Input: part model. Units: mm. Frame: model coordinates. A direction names the side the tool comes from. Coordinates: 2 decimals unless noted, no trailing zeros. Write each loop counter-clockwise with the first axis right and the second up, starting at its lowest first coordinate (ties: lowest second). Pieces come first, ordered by that corner, then holes. Notation, with made-up numbers: (10.5, -17.5) -> (52.5, -17.5) arc R7 cw to (52.5, -7.5) -> close; hole circle Ø9 at (36.5, 76.25). An arc over 180 degrees is marked (long way). Use one line per item in the form item = value. Start each with the question number.
(1) Cut plane D-D on y = 1.25. Return the cut outline in (x, z), plus the area to 3 significant figures.
(2) First-contact query: pin 1 (1 mm diameter, centred on y = -0.5, z = -0.5, fed in from -X); pin 2 (2 mm diameter, centred on y = -0.5, z = -1, fed in from +X). Flat tips, straight axial feed; report the tip coordinate or a pass-through.
(3) Pull-direction query (Y, two-part tool) for faces 1 (the face through (4, 0, -1.7)), 2 (the face through (1.5, -2.25, 0.5)), 3 (the face through (3, 1.75, 1)), 4 (the face through (2, 0, -2)); classes: released by +Y, released by -Y, zero draft, split by the parting line, or undercut.
(4) Cut plane C-C on x = 0.5. Return the cut outline in (y, z).
(5) Ray query, line 1 along Y through (x, z) = (2.05, 1.4); line 2 along Z through (x, y) = (2, 2); line 3 along Z through (x, y) = (3.15, -1.5). Return the intervals inside material, ascending.
(6) Cut plane B-B on x = 5.2. Return the cut outline in (y, z).
(7) Cut plane A-A on z = 0. State how many separate pieces and enclosed holes the cut face has, plus the area to 3 significant figures.
(8) Set-up query: faces 5 (the face through (1.2, 2, 0.6)), 6 (the face through (2, 0, 1.5)), 7 (the face through (1.5, -4.2, 0)). Return all of +Z, -Z, +X, -X, +Y, -Y with unobstructed straight access to the full face (end or side cutting, diameter ignored); none if empty.
```python
from build123d import *

# Parameters (mm, degrees)
SKETCH1_W               = 4
SKETCH1_H               = 4.5
SKETCH1_W_2             = 3
SKETCH1_H_2             = 3.5
BOSS_EXTRUDE1_DEPTH     = 4
SKETCH2_R               = 0.5
BOSS_EXTRUDE2_DEPTH     = 4.55
FILLET1_R               = 0.5
SKETCH3_R               = 1
CUT_EXTRUDE1_DEPTH      = 2.55
BOSS_EXTRUDE3_START     = -0.5
BOSS_EXTRUDE3_DEPTH     = 3
CUT_EXTRUDE2_DEPTH      = 1.5
SKETCH7_W               = 0.349986897
SKETCH7_H               = 2
CUT_EXTRUDE3_DEPTH      = 4.5
CUT_EXTRUDE3_DEPTH_BACK = 7.5


with BuildPart() as part:
    # Sketch1 → Boss-Extrude1 (new body)
    with BuildSketch(Plane(origin=(0, 0, 0), x_dir=(0, 0, -1), z_dir=(1, 0, 0))):
        Rectangle(SKETCH1_W, SKETCH1_H)
        Rectangle(SKETCH1_W_2, SKETCH1_H_2, mode=Mode.SUBTRACT)
    extrude(amount=BOSS_EXTRUDE1_DEPTH)

    # Sketch2 → Boss-Extrude2 (add)
    with BuildSketch(Plane.XZ.offset(2.25)):
        with Locations((2, 0)):
            Circle(SKETCH2_R)
    extrude(amount=BOSS_EXTRUDE2_DEPTH)

    # Fillet1
    fillet1_edges = [part.edges().sort_by_distance(p)[0] for p in [
        (1.5, -6.8, 0),
    ]]
    fillet(fillet1_edges, radius=FILLET1_R)

    # Sketch3 → Cut-Extrude1 (cut)
    with BuildSketch(Plane(origin=(0, 2.25, 0), x_dir=(1, 0, 0), z_dir=(0, 1, 0))):
        with Locations((2, 0)):
            Circle(SKETCH3_R)
    extrude(amount=-CUT_EXTRUDE1_DEPTH, mode=Mode.SUBTRACT)

    # Sketch5 → Boss-Extrude3 (add)
    with BuildSketch(Plane.XY.offset(2).offset(BOSS_EXTRUDE3_START)):
        with BuildLine():
            Line((4, 2.25), (4.403883865, 2.25))
            ThreePointArc((4.403883865, 2.25), (4.586458051, 2.215474668), (4.743818499, 2.116666667))
            Line((4.743818499, 2.116666667), (5.813186883, 1.125261165))
            ThreePointArc((5.813186883, 1.125261165), (5.973243782, 0.755684806), (5.808896382, 0.387996313))
            Line((5.808896382, 0.387996313), (4.596439486, -0.710104164))
            ThreePointArc((4.596439486, -0.710104164), (4.344752484, -0.832406779), (4.066768671, -0.800324431))
            Line((4.066768671, -0.800324431), (1.595431684, 0.240227029))
            Line((1.595431684, 0.240227029), (1.595431684, 0.359579889))
            Line((1.595431684, 0.359579889), (4.04486832, -0.671750473))
            ThreePointArc((4.04486832, -0.671750473), (4.322852132, -0.703832821), (4.574539135, -0.581530206))
            Line((4.574539135, -0.581530206), (5.646078544, 0.388943829))
            ThreePointArc((5.646078544, 0.388943829), (5.810425944, 0.756632322), (5.650369044, 1.126208681))
            Line((5.650369044, 1.126208681), (4.743818499, 1.966666667))
            ThreePointArc((4.743818499, 1.966666667), (4.586458051, 2.065474668), (4.403883865, 2.1))
            Line((4.403883865, 2.1), (4, 2.1))
            Line((4, 2.1), (4, 2.25))
        make_face()
    extrude(amount=-BOSS_EXTRUDE3_DEPTH)

    # Sketch6 → Cut-Extrude2 (cut)
    with BuildSketch(Plane(origin=(0, 2.25, 0), x_dir=(1, 0, 0), z_dir=(0, 1, 0))):
        Polygon((4, 1.5), (5.973252249, 1.15), (5.973252249, 1.5), align=None)
        Polygon((4, -1.5), (5.973252249, -1.15), (5.973252249, -1.5), align=None)
    extrude(amount=-CUT_EXTRUDE2_DEPTH, mode=Mode.SUBTRACT)

    # Sketch7 → Cut-Extrude3 (cut, two sides)
    with BuildSketch(Plane(origin=(4, 0, 0), x_dir=(0, 0, -1), z_dir=(1, 0, 0))) as cut_extrude3_sk:
        with Locations((-1.325006552, -0.25)):
            Rectangle(SKETCH7_W, SKETCH7_H)
        with Locations((1.325006552, -0.25)):
            Rectangle(SKETCH7_W, SKETCH7_H)
    extrude(amount=CUT_EXTRUDE3_DEPTH, mode=Mode.SUBTRACT)
    extrude(cut_extrude3_sk.sketch, amount=-CUT_EXTRUDE3_DEPTH_BACK, mode=Mode.SUBTRACT)


solid = part.part
```
Values:
q1.outline = (0, -2) -> (4, -2) -> (4, -1.5) -> (0, -1.5) -> close; (0, 1.5) -> (4, 1.5) -> (4, 2) -> (0, 2) -> close; (5.52, -1.23) -> (5.68, -1.2) -> (5.68, 1.2) -> (5.52, 1.23) -> close
q1.area = 4.39 mm2
q2.pin_1 = 2.17
q2.pin_2 = 5.9
q3.face_1 = undercut
q3.face_2 = released by -Y
q3.face_3 = undercut
q3.face_4 = zero draft
q4.outline = (-2.25, -2) -> (2.25, -2) -> (2.25, 2) -> (-2.25, 2) -> close; hole (-1.75, -1.5) -> (1.75, -1.5) -> (1.75, 1.5) -> (-1.75, 1.5) -> close
q5.line_1 = -2.25 to -1.75, 1.75 to 2.25
q5.line_2 = -2 to -1, 1 to 2
q5.line_3 = -2 to -1.5, 1.5 to 2
q6.outline = (-0.16, -1.15) -> (-0.02, -1.15) -> (-0.02, 1.15) -> (-0.16, 1.15) -> close; (1.54, -1.29) -> (1.69, -1.29) -> (1.69, 1.29) -> (1.54, 1.29) -> close
q7.separate_pieces = 3
q7.enclosed_holes = 0
q7.area = 8.36 mm2
q8.face_5 = +Y
q8.face_6 = +X, -X
q8.face_7 = -Y
